Geometry: final body of the model. Coordinates: model frame, mm. A direction names the side the tool comes from. Give positions to 0.01 mm unless a question says otherwise; leave off trailing zeros. Write each loop counter-clockwise with the first axis right and the second up, starting at its lowest first coordinate (ties: lowest second). Pieces come first, ordered by that corner, then holes. Notation, with made-up numbers: (21.25, 61.25) -> (59.25, 61.25) arc R10 ccw to (59.25, 70.25) -> close; hole circle Ø8 at (74.25, 62.25). An arc over 180 degrees is marked (long way). Answer as a JSON object with one key per item and string values.
from build123d import *

# Parameters (mm, degrees)
SKETCH_1_W             = 60
SKETCH_1_H             = 30
EXTRUDE_1_DEPTH        = 15
SKETCH_2_W             = 58.8
SKETCH_2_H             = 28.8
CUT_EXTRUDE_2_DEPTH    = 1.5
SKETCH_4_W             = 57
SKETCH_4_H             = 27
CUT_EXTRUDE_3_DEPTH    = 12
SKETCH_5_W             = 44
SKETCH_5_H             = 1
CUT_EXTRUDE_4_DEPTH    = 0.5
EXTRUDE_START          = -5.5
EXTRUDE_4_DEPTH        = 19
MIRROR_START           = -5.5
MIRROR_3_COPY_1_DEPTH  = 19
EXTRUDE_5_DEPTH        = 2
PATTERN_LINEAR_1_COUNT = 4
PATTERN_LINEAR_1_PITCH = 15
CUT_EXTRUDE_5_DEPTH    = 67.001893912
FILLET_1_R             = 0.2
FILLET_2_R             = 0.1


with BuildPart() as part:
    # 草图1 → 凸台-拉伸1 (new body)
    with BuildSketch(Plane(origin=(0, 0, 0), x_dir=(1, 0, 0), z_dir=(0, 1, 0))):
        Rectangle(SKETCH_1_W, SKETCH_1_H)
    extrude(amount=EXTRUDE_1_DEPTH)

    # 草图2 → 切除-拉伸2 (cut)
    with BuildSketch(Plane(origin=(0, 15, 0), x_dir=(1, 0, 0), z_dir=(0, 1, 0))):
        Rectangle(SKETCH_2_W, SKETCH_2_H)
    extrude(amount=-CUT_EXTRUDE_2_DEPTH, mode=Mode.SUBTRACT)

    # 草图4 → 切除-拉伸3 (cut)
    with BuildSketch(Plane(origin=(0, 13.5, 0), x_dir=(1, 0, 0), z_dir=(0, 1, 0))):
        Rectangle(SKETCH_4_W, SKETCH_4_H)
    extrude(amount=-CUT_EXTRUDE_3_DEPTH, mode=Mode.SUBTRACT)

    # 草图5 → 切除-拉伸4 (cut)
    with BuildSketch(Plane.XY.offset(-14.4)):
        with Locations((0, 14)):
            Rectangle(SKETCH_5_W, SKETCH_5_H)
    cut_extrude_4 = extrude(amount=-CUT_EXTRUDE_4_DEPTH, mode=Mode.SUBTRACT)

    # 镜向1: 切除-拉伸4 across plane
    add(cut_extrude_4.mirror(Plane.XY), mode=Mode.SUBTRACT)

    # 草图6 → 凸台-拉伸4 (add)
    with BuildSketch(Plane.XY.offset(15).offset(EXTRUDE_START)):
        with BuildLine():
            Line((30, 7.5), (30, 9))
            Line((30, 9), (30.677124344, 9))
            ThreePointArc((30.677124344, 9), (31.088161527, 9.280042303), (31.555590279, 9.45))
            Line((31.555590279, 9.45), (32.5, 9.45))
            Line((32.5, 9.45), (32.5, 8.943375673))
            Line((32.5, 8.943375673), (30, 7.5))
        make_face()
    extrude_4 = extrude(amount=-EXTRUDE_4_DEPTH)

    # 镜向2: 凸台-拉伸4 across plane
    add(extrude_4.mirror(Plane(origin=(0, 7.5, 0), x_dir=(0, 0, 1), z_dir=(0, -1, 0))))

    # 镜向3: 凸台-拉伸4 across plane
    add(extrude_4.mirror(Plane(origin=(0, 0, 0), x_dir=(0, 0, 1), z_dir=(1, 0, 0))))

    # 镜向3 copy 1 sketch → 镜向3 copy 1 (add)
    with BuildSketch(Plane(origin=(0, 15, 15), x_dir=(-1, 0, 0), z_dir=(0, 0, 1)).offset(MIRROR_START)):
        with BuildLine():
            Line((30, 7.5), (30, 9))
            Line((30, 9), (30.677124344, 9))
            ThreePointArc((30.677124344, 9), (31.088161527, 9.280042303), (31.555590279, 9.45))
            Line((31.555590279, 9.45), (32.5, 9.45))
            Line((32.5, 9.45), (32.5, 8.943375673))
            Line((32.5, 8.943375673), (30, 7.5))
        make_face()
    extrude(amount=-MIRROR_3_COPY_1_DEPTH)

    # 草图7 → 凸台-拉伸5 (add, symmetric)
    with BuildSketch(Plane.XY):
        with BuildLine():
            Line((-24, 0), (-21, 0))
            Line((-21, 0), (-21, -0.677124344))
            ThreePointArc((-21, -0.677124344), (-20.719957697, -1.088161527), (-20.55, -1.555590279))
            Line((-20.55, -1.555590279), (-20.55, -2.5))
            Line((-20.55, -2.5), (-24.45, -2.5))
            Line((-24.45, -2.5), (-24.45, -1.555590279))
            ThreePointArc((-24.45, -1.555590279), (-24.280042303, -1.088161527), (-24, -0.677124344))
            Line((-24, -0.677124344), (-24, 0))
        make_face()
    extrude_5 = extrude(amount=EXTRUDE_5_DEPTH, both=True)

    # 阵列(线性)1: 凸台-拉伸5 ×4
    with Locations(*[(i * PATTERN_LINEAR_1_PITCH, 0, 0) for i in range(1, PATTERN_LINEAR_1_COUNT)]):
        add(extrude_5)

    # 草图8 → 切除-拉伸5 (cut, through all)
    with BuildSketch(Plane.ZY.offset(30)):
        with BuildLine():
            Line((1.5, 0), (1.5, -0.677124344))
            ThreePointArc((1.5, -0.677124344), (1.780042303, -1.088161527), (1.95, -1.555590279))
            Line((1.95, -1.555590279), (1.95, -2.5))
            Line((1.95, -2.5), (2, -2.5))
            Line((2, -2.5), (2, 0))
            Line((2, 0), (1.5, 0))
        make_face()
        with BuildLine():
            Line((-2, 0), (-1.5, 0))
            Line((-1.5, 0), (-1.5, -0.677124344))
            ThreePointArc((-1.5, -0.677124344), (-1.780042303, -1.088161527), (-1.95, -1.555590279))
            Line((-1.95, -1.555590279), (-1.95, -2.5))
            Line((-1.95, -2.5), (-2, -2.5))
            Line((-2, -2.5), (-2, 0))
        make_face()
    extrude(amount=-CUT_EXTRUDE_5_DEPTH, mode=Mode.SUBTRACT)

    # 圆角1
    fillet_1_edges = [part.edges().sort_by_distance(p)[0] for p in [
        (0, 15, 15),
        (30, 15, 0),
        (0, 15, -15),
        (30, 0, 0),
        (0, 0, 15),
        (-30, 0, 0),
        (0, 0, -15),
        (-30, 15, 0),
        (30, 7.5, -15),
        (30, 7.5, 15),
        (-30, 7.5, 15),
        (-30, 7.5, -15),
    ]]
    fillet(fillet_1_edges, radius=FILLET_1_R)

    # 圆角2
    fillet_2_edges = [part.edges().sort_by_distance(p)[0] for p in [
        (-32.5, 9.45, 0),
        (-32.5, 9.196687836, -9.5),
        (-32.5, 6.056624327, 0),
        (-32.5, 5.803312164, -9.5),
        (-32.5, 5.55, 0),
        (-32.5, 5.803312164, 9.5),
        (24.45, -2.5, 0),
        (20.55, -2.5, 0),
        (9.45, -2.5, 0),
        (5.55, -2.5, 0),
        (-5.55, -2.5, 0),
        (-9.45, -2.5, 0),
        (-20.55, -2.5, 0),
        (-24.45, -2.5, 0),
        (-22.5, -2.5, -1.95),
        (-7.5, -2.5, -1.95),
        (7.5, -2.5, -1.95),
        (22.5, -2.5, -1.95),
        (-22.5, -2.5, 1.95),
        (-7.5, -2.5, 1.95),
        (7.5, -2.5, 1.95),
        (22.5, -2.5, 1.95),
        (32.5, 8.943375673, 0),
        (32.5, 9.196687836, -9.5),
        (32.5, 9.45, 0),
        (32.5, 9.196687836, 9.5),
        (32.5, 5.803312164, 9.5),
        (32.5, 6.056624327, 0),
        (32.5, 5.55, 0),
        (32.5, 5.803312164, -9.5),
        (-32.5, 9.196687836, 9.5),
        (-32.5, 8.943375673, 0),
    ]]
    fillet(fillet_2_edges, radius=FILLET_2_R)


solid = part.part
Q1. Mould query, pull axis Z, two halves, no side actions, for faces 5 (the flat face through (29.4, 14, 0)), 6 (the flat face through (-31, 9, -9.5)), 7 (the flat face through (31, 9, 9.5)). Classes: pulls with the +Z half, pulls with the -Z half, needs draft (parallel to the pull), parting line crosses it, or undercut.
Values:
{"face 5": "undercut", "face 6": "pulls with the -Z half", "face 7": "pulls with the +Z half"}
Q2. Cut plane D-D (x = -26.5). Return the cut outline in (y, z), and give its area (3 significant figures).
Values:
{"outline": "(0, -14.8) arc R0.2 ccw to (0.2, -15) -> (14.8, -15) arc R0.2 ccw to (15, -14.8) -> (15, -14.4) -> (13.5, -14.4) -> (13.5, -13.5) -> (1.5, -13.5) -> (1.5, 13.5) -> (13.5, 13.5) -> (13.5, 14.4) -> (15, 14.4) -> (15, 14.8) arc R0.2 ccw to (14.8, 15) -> (0.2, 15) arc R0.2 ccw to (0, 14.8) -> close", "area": "82.8 mm²"}
Q3. Cut plane A-A (y = 11.75). Return the cut outline in (x, z), and give its area (3 significant figures).
Values:
{"outline": "(-30, -14.8) arc R0.2 ccw to (-29.8, -15) -> (29.8, -15) arc R0.2 ccw to (30, -14.8) -> (30, 14.8) arc R0.2 ccw to (29.8, 15) -> (-29.8, 15) arc R0.2 ccw to (-30, 14.8) -> close; hole (-28.5, -13.5) -> (28.5, -13.5) -> (28.5, 13.5) -> (-28.5, 13.5) -> close", "area": "261 mm²"}
Q4. Cut plane C-C (z = 12). Return the cut outline in (x, y).
Values:
{"outline": "(-30, 0.2) arc R0.2 ccw to (-29.8, 0) -> (29.8, 0) arc R0.2 ccw to (30, 0.2) -> (30, 14.8) arc R0.2 ccw to (29.8, 15) -> (29.4, 15) -> (29.4, 13.5) -> (28.5, 13.5) -> (28.5, 1.5) -> (-28.5, 1.5) -> (-28.5, 13.5) -> (-29.4, 13.5) -> (-29.4, 15) -> (-29.8, 15) arc R0.2 ccw to (-30, 14.8) -> close"}
Q5. First-contact query: P1, Ø0.6, axis at y = 14, z = 14.5, coming from the -X side; P2, Ø0.7, axis at x = -32, z = -3.5, coming from the +Y side; P3, Ø4, axis at x = -16, z = 9, coming from the -Y side. Flat tips, straight axial feed; report the tip coordinate or a pass-through.
Values:
{"P1": "x = -30", "P2": "y = 9.45", "P3": "y = 0"}
Q6. Set-up query: faces 1 (the flat face through (0, 13.5, 14)), 2 (the flat face through (-31, 6, 9.5)), 3 (the flat face through (31.242, 6.783, 0.133)), 4 (the flat face through (28.5, 8, 0)). Return all of +Z, -Z, +X, -X, +Y, -Y with unobstructed straight access to the full face (end or side cutting, diameter ignored); none if empty.
Values:
{"face 1": "none", "face 2": "+Z, -X, +Y, -Y", "face 3": "+Z, -Z, +X", "face 4": "+Y"}
Q7. Cut plane B-B (x = -3). Return the cut outline in (y, z).
Values:
{"outline": "(0, -14.8) arc R0.2 ccw to (0.2, -15) -> (14.8, -15) arc R0.2 ccw to (15, -14.8) -> (15, -14.4) -> (14.5, -14.4) -> (14.5, -14.9) -> (13.5, -14.9) -> (13.5, -13.5) -> (1.5, -13.5) -> (1.5, 13.5) -> (13.5, 13.5) -> (13.5, 14.9) -> (14.5, 14.9) -> (14.5, 14.4) -> (15, 14.4) -> (15, 14.8) arc R0.2 ccw to (14.8, 15) -> (0.2, 15) arc R0.2 ccw to (0, 14.8) -> close"}
Q8. Material intervals for L1, parallel to X at y = 5.5, z = -9.75; L2, parallel to Z at x = -1, y = 8.75; L3, parallel to X at y = 14.25, z = 0.5, sorted ascending. Write a range as from..to.
Values:
{"L1": "-30..-28.5, 28.5..30", "L2": "-15..-13.5, 13.5..15", "L3": "-30..-29.4, 29.4..30"}
